from build123d import *

# Parameters (mm, degrees)
F1_DEPTH  = 3
F2_R      = 1.5
F3_DEPTH  = 3.001
F4_R      = 1.6
F5_DEPTH  = 3.001
F6_W      = 40
F6_H      = 3
F7_DEPTH  = 0.5
F8_W      = 23.5
F8_H      = 3
F9_DEPTH  = 0.25
F10_W     = 23.5000022292
F10_H     = 3
F11_DEPTH = 0.25
F12_W     = 23.5000022292
F12_H     = 3
F13_DEPTH = 3


with BuildPart() as f1:
    # F0 (on Top) → F1 (new body)
    with BuildSketch(Plane.XY):
        Polygon((30, -30), (30, 30), (-30, 30), (-30, -30), (-20, -30), (-20, -15.5000011146), (-19.9802070856, -13.5000011146), (-10, -13.5000011146), (-10, -7.5000011146), (-20, -7.5000011146), (-20, 15.4999988854), (20, 15.5000011146), (20, -7.5000011146), (10, -7.5000011146), (10, -13.5000011146), (20, -13.5000011146), (20, -15.4999988854), (20, -30), align=None)
        with BuildLine():
            Line((-20, -15.5000011146), (-20, -30))
            ThreePointArc((-20, -30), (-17.3048696173, -20.3531097858), (-10, -13.5000011146))
            Line((-10, -13.5000011146), (-19.9802070856, -13.5000011146))
            Line((-19.9802070856, -13.5000011146), (-20, -15.5000011146))
        make_face()
        with BuildLine():
            ThreePointArc((10, -13.5000011146), (17.3048696173, -20.3531097858), (20, -30))
            Line((20, -30), (20, -15.4999988854))
            Line((20, -15.4999988854), (20, -13.5000011146))
            Line((20, -13.5000011146), (10, -13.5000011146))
        make_face()
    extrude(amount=F1_DEPTH)

    # F2 (on face) → F3 (cut, through all)
    with BuildSketch(Plane.XY.offset(3)):
        with Locations((-25, 23)):
            Circle(F2_R)
        with Locations((25, 23)):
            Circle(F2_R)
        with Locations((-25, -23)):
            Circle(F2_R)
        with Locations((25, -23)):
            Circle(F2_R)
    extrude(amount=-F3_DEPTH, mode=Mode.SUBTRACT)

    # F4 (on face) → F5 (cut, through all)
    with BuildSketch(Plane.XY.offset(3)):
        with Locations((25, -17)):
            Circle(F4_R)
        with Locations((-25, -17)):
            Circle(F4_R)
        with Locations((0, 23)):
            Circle(F4_R)
    extrude(amount=-F5_DEPTH, mode=Mode.SUBTRACT)

    # F6 (on face) → F7 (cut)
    with BuildSketch(Plane(origin=(-8.638e-07, 15.5, 0), x_dir=(1, 5.57e-08, 0), z_dir=(5.57e-08, -1, 0))):
        with Locations((8.638e-07, 1.5)):
            Rectangle(F6_W, F6_H)
    extrude(amount=-F7_DEPTH, mode=Mode.SUBTRACT)

    # F8 (on face) → F9 (cut)
    with BuildSketch(Plane.YZ.offset(-20)):
        with Locations((4.2499988854, 1.5)):
            Rectangle(F8_W, F8_H)
    extrude(amount=-F9_DEPTH, mode=Mode.SUBTRACT)

    # F10 (on face) → F11 (cut)
    with BuildSketch(Plane(origin=(20, 0, 0), x_dir=(0, -1, 0), z_dir=(-1, 0, 0))):
        with Locations((-4.25, 1.5)):
            Rectangle(F10_W, F10_H)
    extrude(amount=-F11_DEPTH, mode=Mode.SUBTRACT)

    # F12 (on face) → F13 (cut)
    with BuildSketch(Plane(origin=(20.25, 0, 0), x_dir=(0, -1, 0), z_dir=(-1, 0, 0))):
        with Locations((-4.25, 1.5)):
            Rectangle(F12_W, F12_H)
    extrude(amount=-F13_DEPTH, mode=Mode.SUBTRACT)


solid = f1.part
Source: CAD feature listing. Evaluate the final solid. Frame: model axes, mm. A direction names the side the tool comes from. Round coordinates to 2 decimals unless told otherwise and drop trailing zeros. Loops run counter-clockwise (first coordinate to the right, second up) from the corner with the lowest first, then second, coordinate; pieces in that order, holes last.
Q1. Section D-D, the plane y = 23. Return loops of the section in (x, z), plus the area to 3 significant figures.
Q2. First-contact query: P1, Ø1, axis at x = 17.5, z = 1, coming from the -Y side. Flat tip, straight axial feed; report the tip coordinate or a pass-through.
Q3. Ray query, line 1 (Y direction, x = 25, z = 0.95); line 2 (X direction, y = 0, z = 1); line 3 (Y direction, x = 2.5, z = 0.6). Return the intervals inside material, ascending.
Q4. Section A-A, the plane y = 7. Return loops of the section in (x, z).
Q5. Section C-C, the plane x = -25. Return loops of the section in (y, z), plus the area to 3 significant figures.
Q6. Access query for faces 1 (the face through (-10, -11, 1)), 2 (the face through (23.25, 4, 2)), 3 (the face through (25, -30, 1)). Directions: +Z, -Z, +X, -X, +Y, -Y. A direction counts if a zero-diameter tool reaches every point of the face in a straight line with its end or side. Return the directions, or none.
Q7. Section B-B, the plane z = 1.6. State how many separate pieces and enclosed holes the cut face has, plus the area to 3 significant figures.
Solutions:
1. outline: (-30, 0) - (-26.5, 0) - (-26.5, 3) - (-30, 3) - close; (-23.5, 0) - (-1.6, 0) - (-1.6, 3) - (-23.5, 3) - close; (1.6, 0) - (23.5, 0) - (23.5, 3) - (1.6, 3) - close; (26.5, 0) - (30, 0) - (30, 3) - (26.5, 3) - close
1. area: 152 mm2
2. P1: stops at y = -21.61
3. line 1: y = -30 to -24.5, -21.5 to -18.6, -15.4 to 21.5, 24.5 to 30
3. line 2: x = -30 to -20.25, 23.25 to 30
3. line 3: y = 16 to 30
4. outline: (-30, 0) - (-20.25, 0) - (-20.25, 3) - (-30, 3) - close; (23.25, 0) - (30, 0) - (30, 3) - (23.25, 3) - close
5. outline: (-30, 0) - (-24.5, 0) - (-24.5, 3) - (-30, 3) - close; (-21.5, 0) - (-18.6, 0) - (-18.6, 3) - (-21.5, 3) - close; (-15.4, 0) - (21.5, 0) - (21.5, 3) - (-15.4, 3) - close; (24.5, 0) - (30, 0) - (30, 3) - (24.5, 3) - close
5. area: 152 mm2
6. face 1: +Z, -Z, -Y
6. face 2: +Z, -Z
6. face 3: +Z, -Z, +X, -X, -Y
7. separate pieces: 1
7. enclosed holes: 7
7. area: 1,840 mm2
